Geometry: see drawing. Coordinates: mm, zero at the bounding-box minimum. Coordinates: 2 decimals unless noted, no trailing zeros. Write each loop counter-clockwise with the first axis right and the second up, starting at its lowest first coordinate (ties: lowest second). Pieces come first, ordered by that corner, then holes. Notation, with made-up numbers: (-4.75, 69) - (7.25, 69) arc R27 cw to (7.25, 106) - close; hole circle Ø5 at (-8.75, 50). An arc over 180 degrees is marked (long way). Use CSV: the item, a comma, the result in double quotes.
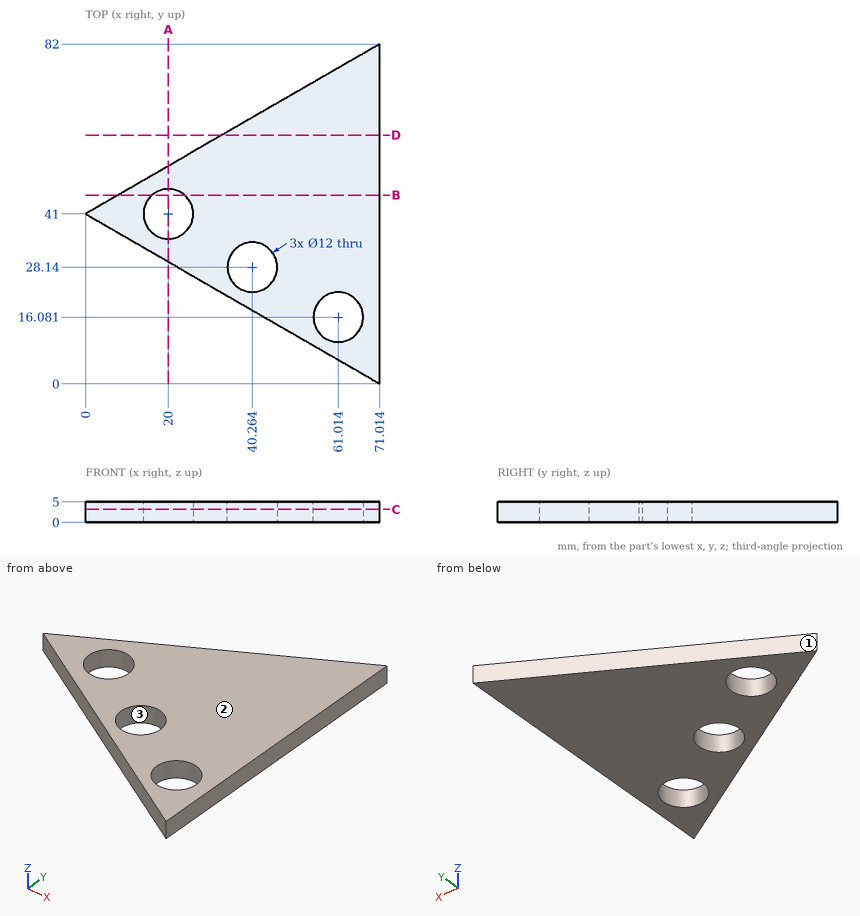
(1) Cut plane C-C on z = 3.15. Return loops of the section in (x, y), and give its area (3 significant figures).
Check values:
outline,"(0, 41) - (71.01, 0) - (71.01, 82) - close; hole circle Ø12 at (20, 41); hole circle Ø12 at (40.26, 28.14); hole circle Ø12 at (61.01, 16.08)"
area,"2,570 mm^2"
(2) Pin query (flat end, axial travel): pin 1 Ø8 at (x, y) = (19, 53.5) entering from +Z; pin 2 Ø1 at (x, z) = (36.5, 3.5) entering from -Y; pin 3 Ø2 at (x, z) = (52, 4) entering from -Y. Return the tip coordinate at first contact, or that it passes through.
Check values:
pin 1,"z = 5"
pin 2,"y = 19.64"
pin 3,"y = 10.4"
(3) Ray query, probe 1 along Y at (x, z) = (20.5, 3.2) (1 decimal); probe 2 along Y at (x, z) = (58, 4.6); probe 3 along X at (y, z) = (40, 0.7) (1 decimal). Return the intervals inside material, ascending. Write a range as from..to.
Check values:
probe 1,"29.2..35, 47..52.8"
probe 2,"7.51..10.89, 21.27..74.49"
probe 3,"1.7..14.1, 25.9..71"
(4) Draft query along X for the marked faces 1, 2 and 3. Return one class per face: pulls with the +X half, pulls with the -X half, needs draft (parallel to the pull), parting line crosses it, or undercut.
Check values:
face 1,"pulls with the -X half"
face 2,"needs draft"
face 3,"undercut"
(5) Cut plane A-A on x = 20. Return loops of the section in (y, z).
Check values:
outline,"(29.45, 0) - (35, 0) - (35, 5) - (29.45, 5) - close; (47, 0) - (52.55, 0) - (52.55, 5) - (47, 5) - close"
(6) Cut plane B-B on y = 45.5. Return loops of the section in (x, z).
Check values:
outline,"(7.79, 0) - (16.03, 0) - (16.03, 5) - (7.79, 5) - close; (23.97, 0) - (71.01, 0) - (71.01, 5) - (23.97, 5) - close"
(7) Cut plane D-D on y = 60. Return loops of the section in (x, z).
Check values:
outline,"(32.91, 0) - (71.01, 0) - (71.01, 5) - (32.91, 5) - close"
